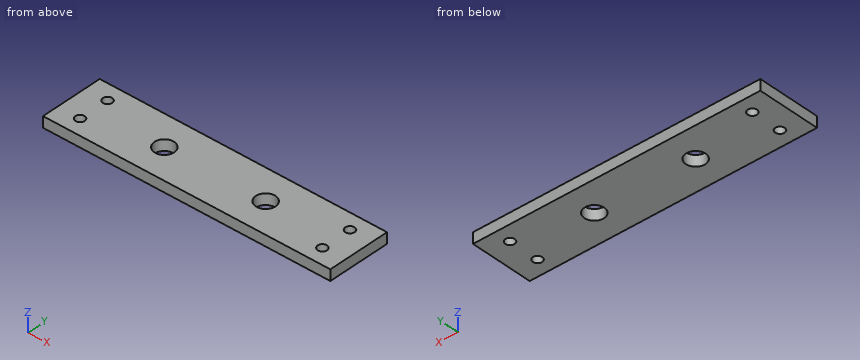
```python
from build123d import *

# Parameters (mm, degrees)
SKETCH1_W           = 160
SKETCH1_H           = 35
BOSS_EXTRUDE1_DEPTH = 6
CUT_EXTRUDE1_REACH  = 84.111
SKETCH2_R           = 2.6
CUT_EXTRUDE2_REACH  = 84.111
SKETCH3_R           = 5.5


with BuildPart() as part:
    # Sketch1 → Boss-Extrude1 (new body)
    with BuildSketch(Plane.XY):
        Rectangle(SKETCH1_W, SKETCH1_H)
    extrude(amount=BOSS_EXTRUDE1_DEPTH)

    # Sketch2 → Cut-Extrude1 (cut, up to next)
    with BuildSketch(Plane.XY.offset(6), mode=Mode.PRIVATE) as cut_extrude1_sk1:
        with Locations((67.5, 8.5)):
            Circle(SKETCH2_R)
    cut_extrude1_tool1 = extrude(cut_extrude1_sk1.sketch, amount=-CUT_EXTRUDE1_REACH, mode=Mode.PRIVATE) & part.part
    # Sketch2 → Cut-Extrude1 (cut, up to next)
    with BuildSketch(Plane.XY.offset(6), mode=Mode.PRIVATE) as cut_extrude1_sk2:
        with Locations((67.5, -8.5)):
            Circle(SKETCH2_R)
    cut_extrude1_tool2 = extrude(cut_extrude1_sk2.sketch, amount=-CUT_EXTRUDE1_REACH, mode=Mode.PRIVATE) & part.part
    # Sketch2 → Cut-Extrude1 (cut, up to next)
    with BuildSketch(Plane.XY.offset(6), mode=Mode.PRIVATE) as cut_extrude1_sk3:
        with Locations((-67.5, 8.5)):
            Circle(SKETCH2_R)
    cut_extrude1_tool3 = extrude(cut_extrude1_sk3.sketch, amount=-CUT_EXTRUDE1_REACH, mode=Mode.PRIVATE) & part.part
    # Sketch2 → Cut-Extrude1 (cut, up to next)
    with BuildSketch(Plane.XY.offset(6), mode=Mode.PRIVATE) as cut_extrude1_sk4:
        with Locations((-67.5, -8.5)):
            Circle(SKETCH2_R)
    cut_extrude1_tool4 = extrude(cut_extrude1_sk4.sketch, amount=-CUT_EXTRUDE1_REACH, mode=Mode.PRIVATE) & part.part
    add(cut_extrude1_tool1.solids().sort_by_distance((67.5, 8.5, 6))[0], mode=Mode.SUBTRACT)
    add(cut_extrude1_tool2.solids().sort_by_distance((67.5, -8.5, 6))[0], mode=Mode.SUBTRACT)
    add(cut_extrude1_tool3.solids().sort_by_distance((-67.5, 8.5, 6))[0], mode=Mode.SUBTRACT)
    add(cut_extrude1_tool4.solids().sort_by_distance((-67.5, -8.5, 6))[0], mode=Mode.SUBTRACT)

    # Sketch3 → Cut-Extrude2 (cut, up to next)
    with BuildSketch(Plane.XY.offset(6), mode=Mode.PRIVATE) as cut_extrude2_sk1:
        with Locations((28.22, 0)):
            Circle(SKETCH3_R)
    cut_extrude2_tool1 = extrude(cut_extrude2_sk1.sketch, amount=-CUT_EXTRUDE2_REACH, mode=Mode.PRIVATE) & part.part
    # Sketch3 → Cut-Extrude2 (cut, up to next)
    with BuildSketch(Plane.XY.offset(6), mode=Mode.PRIVATE) as cut_extrude2_sk2:
        with Locations((-28.22, 0)):
            Circle(SKETCH3_R)
    cut_extrude2_tool2 = extrude(cut_extrude2_sk2.sketch, amount=-CUT_EXTRUDE2_REACH, mode=Mode.PRIVATE) & part.part
    add(cut_extrude2_tool1.solids().sort_by_distance((28.22, 0, 6))[0], mode=Mode.SUBTRACT)
    add(cut_extrude2_tool2.solids().sort_by_distance((-28.22, 0, 6))[0], mode=Mode.SUBTRACT)


solid = part.part
```
Design review of the part built by this model. Coordinates are the model's own, in mm. Coordinates: 2 decimals unless noted, no trailing zeros. Write each loop counter-clockwise with the first axis right and the second up, starting at its lowest first coordinate (ties: lowest second). Pieces come first, ordered by that corner, then holes. Notation, with made-up numbers: M 56,15 L 65,15 A23 ccw 65,45 Z; hole C 66,-33.5 d5. An arc over 180 degrees is marked long. Answer as a JSON object with one key per item and string values.
Item 1: Add section C-C, the plane z = 1.05. Give the boundary of the cut face in (x, y), and give its area (4 significant figures).
Outcome:
{"outline": "M -80,-17.5 L 80,-17.5 L 80,17.5 L -80,17.5 Z; hole C -67.5,-8.5 d5.2; hole C -67.5,8.5 d5.2; hole C -28.22,0 d11; hole C 28.22,0 d11; hole C 67.5,-8.5 d5.2; hole C 67.5,8.5 d5.2", "area": "5,325 mm²"}
Item 2: Insertion check: pin 1 Ø10 at (x, y) = (-28.22, 0) entering from -Z. The pin has a flat end and moves straight along its axis. Give the tip position at first contact, or say it passes through.
Outcome:
{"pin 1": "through"}
Item 3: Add section B-B, the plane x = 28.22. Give the boundary of the cut face in (y, z), and give its area (3 significant figures).
Outcome:
{"outline": "M -17.5,0 L -5.5,0 L -5.5,6 L -17.5,6 Z; M 5.5,0 L 17.5,0 L 17.5,6 L 5.5,6 Z", "area": "144 mm²"}
Item 4: Add section A-A, the plane y = 8.5. Give the boundary of the cut face in (x, z), and give its area (3 significant figures).
Outcome:
{"outline": "M -80,0 L -70.1,0 L -70.1,6 L -80,6 Z; M -64.9,0 L 64.9,0 L 64.9,6 L -64.9,6 Z; M 70.1,0 L 80,0 L 80,6 L 70.1,6 Z", "area": "898 mm²"}
Item 5: Add section D-D, the plane x = 67.5. Give the boundary of the cut face in (y, z).
Outcome:
{"outline": "M -17.5,0 L -11.1,0 L -11.1,6 L -17.5,6 Z; M -5.9,0 L 5.9,0 L 5.9,6 L -5.9,6 Z; M 11.1,0 L 17.5,0 L 17.5,6 L 11.1,6 Z"}
Item 6: Wall thickness on probe 1 along Y at (x, z) = (-67.5, 1.9); probe 2 along Y at (x, z) = (28.22, 3.35); probe 3 along X at (y, z) = (7, 0.9): over which ranges is each line inside the solid? List them lowest first.
Outcome:
{"probe 1": "-17.5 to -11.1, -5.9 to 5.9, 11.1 to 17.5", "probe 2": "-17.5 to -5.5, 5.5 to 17.5", "probe 3": "-80 to -69.62, -65.38 to 65.38, 69.62 to 80"}
